Can you work these out from the model? Positions are in its coordinate system, mm. Face numbers are marked on the shaded views. Give positions to 0.01 mm unless a question says otherwise; leave off trailing zeros. Loops run counter-clockwise (first coordinate to the right, second up) from the corner with the lowest first, then second, coordinate; pieces in that order, holes last. Notation, with made-up numbers: M -9.5,39.5 L -2.5,39.5 A11 cw -2.5,43.5 Z; hole C 84.25,85.25 d2. An arc over 180 degrees is marked long. One line per item, written item: value. Start each with the question number.
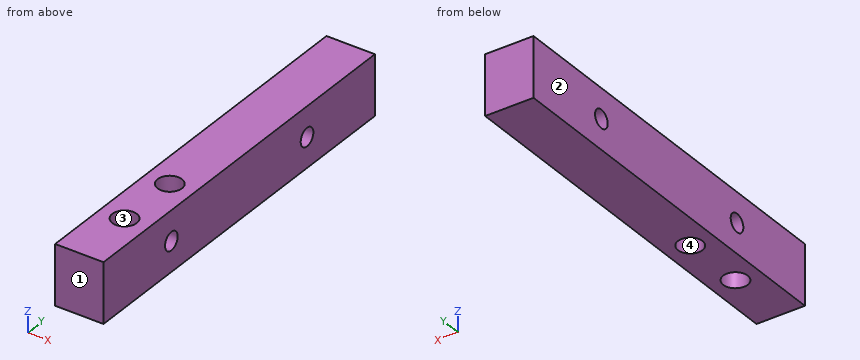
from build123d import *

# Parameters (mm, degrees)
SKETCH1_W           = 9.525
SKETCH1_H           = 76.2
BOSS_EXTRUDE1_DEPTH = 11.811
SKETCH2_R           = 1.778
CUT_EXTRUDE1_DEPTH  = 10.525
SKETCH3_R           = 2.413
CUT_EXTRUDE2_DEPTH  = 12.811


with BuildPart() as part:
    # Sketch1 → Boss-Extrude1 (new body)
    with BuildSketch(Plane.XY):
        with Locations((4.7625, 38.1)):
            Rectangle(SKETCH1_W, SKETCH1_H)
    extrude(amount=BOSS_EXTRUDE1_DEPTH)

    # Sketch2 → Cut-Extrude1 (cut, through all)
    with BuildSketch(Plane.ZY):
        with Locations((5.9055, 57.15)):
            Circle(SKETCH2_R)
        with Locations((5.9055, 19.05)):
            Circle(SKETCH2_R)
    extrude(amount=-CUT_EXTRUDE1_DEPTH, mode=Mode.SUBTRACT)

    # Sketch3 → Cut-Extrude2 (cut, through all)
    with BuildSketch(Plane(origin=(0, 0, 0), x_dir=(-1, 0, 0), z_dir=(0, 0, -1))):
        with Locations((-4.7625, 25.4)):
            Circle(SKETCH3_R)
        with Locations((-4.7625, 12.7)):
            Circle(SKETCH3_R)
    extrude(amount=-CUT_EXTRUDE2_DEPTH, mode=Mode.SUBTRACT)


solid = part.part
Q1. I need wall thicknesses on line 1 along Y through (x, z) = (6, 10.25); line 2 along Y through (x, z) = (1.25, 7); line 3 along Y through (x, z) = (3.5, 5.25). Which ranges of each line are inside material? Lowest first, please.
Q2. If we section it at D-D, the plane y = 57.15: Write out the boundary of the cut face in (x, z) (1 decimal), plus the area to 3 significant figures.
Q3. If we section it at C-C, the plane x = 8: Write out the boundary of the cut face in (y, z).
Q4. For P1, Ø4, axis at x = 4.76, y = 12.7, coming from the -Z side, with a flat end and sliding along its axis, tell me the tip position at first contact or that it passes through.
Q5. If we mould it in two halves opening along X, with no side actions, what happens to the marked faces 1, 2, 3 and 4? For each: released by +X, released by -X, zero draft, split by the parting line, or undercut.
Q6. If we section it at B-B, the plane z = 5.25: Write out the boundary of the cut face in (x, y) (1 decimal), plus the area to 3 significant figures.
Q7. If we section it at A-A, the plane y = 25.4: Write out the boundary of the cut face in (x, z) (1 decimal), plus the area to 3 significant figures.
Response:
1. line 1: 0 to 10.63, 14.77 to 23.33, 27.47 to 76.2
1. line 2: 0 to 17.65, 20.45 to 55.75, 58.55 to 76.2
1. line 3: 0 to 10.64, 14.76 to 17.4, 20.7 to 23.34, 27.46 to 55.5, 58.8 to 76.2
2. outline: M 0,0 L 9.5,0 L 9.5,4.1 L 0,4.1 Z; M 0,7.7 L 9.5,7.7 L 9.5,11.8 L 0,11.8 Z
2. area: 78.6 mm^2
3. outline: M 0,0 L 76.2,0 L 76.2,11.81 L 0,11.81 Z; hole C 19.05,5.91 d3.56; hole C 57.15,5.91 d3.56
4. P1: through
5. face 1: zero draft
5. face 2: released by -X
5. face 3: undercut
5. face 4: undercut
6. outline: M 0,0 L 9.5,0 L 9.5,17.4 L 0,17.4 Z; M 0,20.7 L 9.5,20.7 L 9.5,55.5 L 0,55.5 Z; M 0,58.8 L 9.5,58.8 L 9.5,76.2 L 0,76.2 Z; hole C 4.8,12.7 d4.8; hole C 4.8,25.4 d4.8
6. area: 626 mm^2
7. outline: M 0,0 L 2.3,0 L 2.3,11.8 L 0,11.8 Z; M 7.2,0 L 9.5,0 L 9.5,11.8 L 7.2,11.8 Z
7. area: 55.5 mm^2
